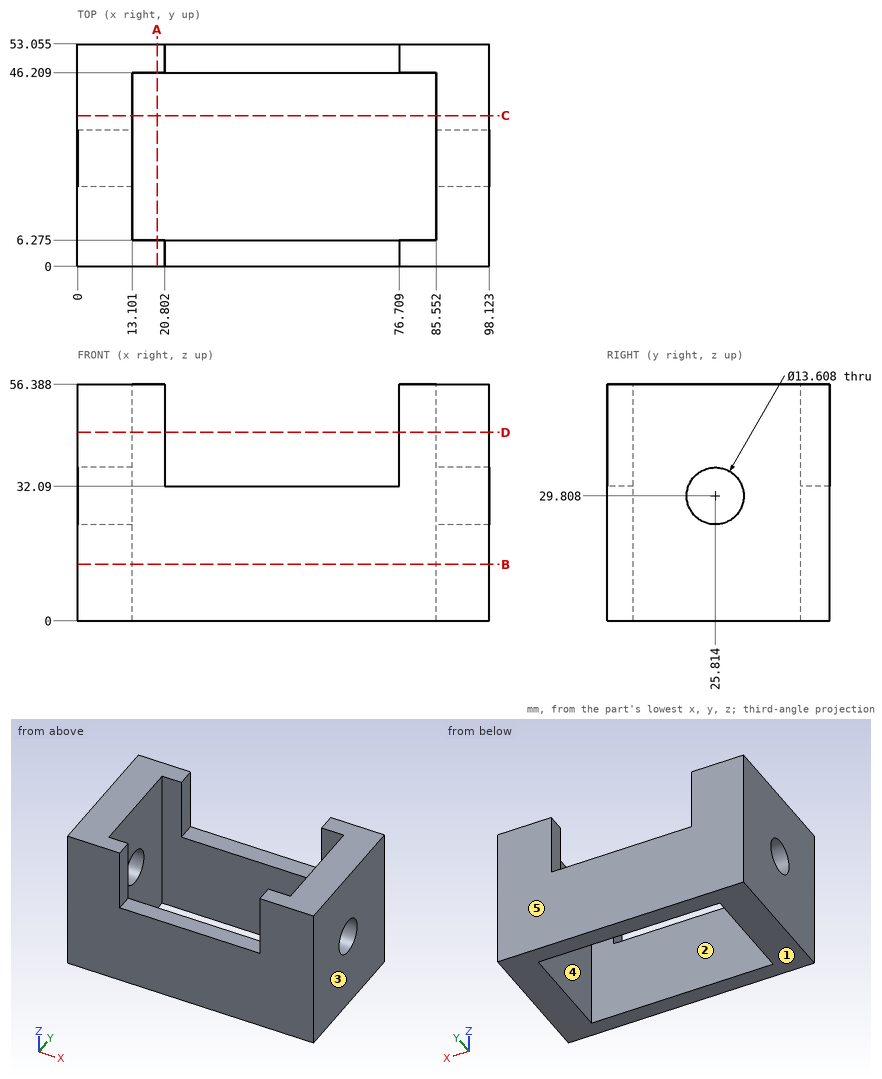
Source: three-view drawing plus pictorial views. Frame: mm from the lowest corner of the part. A direction names the side the tool comes from. Give positions to 0.01 mm unless a question says otherwise; leave off trailing zeros. Write each loop counter-clockwise with the first axis right and the second up, starting at its lowest first coordinate (ties: lowest second). Pieces come first, ordered by that corner, then holes. Notation, with made-up numbers: (-15, 33) -> (4, 33) arc R30 cw to (4, 68) -> close; hole circle Ø2 at (-39, 74.25). An arc over 180 degrees is marked (long way). Write item = value, one per line.
Q1. Mould query, pull axis X, two halves, no side actions, for the marked faces 1, 2 and 3. Classes: +X half, -X half, draft (parallel to the pull), parting line (faces both ways), or undercut.
Here are the results:
face_1 = draft
face_2 = undercut
face_3 = +X half
Q2. Reachability of the marked faces 4 and 5 from +Z, -Z, +X, -X, +Y, -Y: full face, straight path, thin tool, end or side. Return the list, or none.
Here are the results:
face_4 = +Z, -Z
face_5 = +Z, -Z, +X, -X, +Y
Q3. First-contact query: pin 1 (6 mm diameter, centred on x = 37, z = 37.5, fed in from -Y); pin 2 (7.5 mm diameter, centred on x = 54, y = 50.5, fed in from +Z). Flat tips, straight axial feed; report the tip coordinate or a pass-through.
Here are the results:
pin_1 = through
pin_2 = 32.09
Q4. Cut plane C-C on y = 36. Return loops of the section in (x, z).
Here are the results:
outline = (0, 0) -> (13.1, 0) -> (13.1, 56.39) -> (0, 56.39) -> close; (85.55, 0) -> (98.12, 0) -> (98.12, 56.39) -> (85.55, 56.39) -> close
Q5. Line query: line 1 (Y direction, x = 24, z = 15) (1 decimal); line 2 (X direction, y = 19.5, z = 35); line 3 (X direction, y = 49.5, z = 51). Output: solid intervals per line, ascending. Write a range as from..to.
Here are the results:
line_1 = 0..6.3, 46.2..53.1
line_2 = 0..13.1, 85.55..98.12
line_3 = 0..20.8, 76.71..98.12
Q6. Cut plane D-D on z = 45. Return loops of the section in (x, y) (1 decimal).
Here are the results:
outline = (0, 0) -> (20.8, 0) -> (20.8, 6.3) -> (13.1, 6.3) -> (13.1, 46.2) -> (20.8, 46.2) -> (20.8, 53.1) -> (0, 53.1) -> close; (76.7, 0) -> (98.1, 0) -> (98.1, 53.1) -> (76.7, 53.1) -> (76.7, 46.2) -> (85.6, 46.2) -> (85.6, 6.3) -> (76.7, 6.3) -> close
Q7. Cut plane A-A on x = 19. Return loops of the section in (y, z) (1 decimal).
Here are the results:
outline = (0, 0) -> (6.3, 0) -> (6.3, 56.4) -> (0, 56.4) -> close; (46.2, 0) -> (53.1, 0) -> (53.1, 56.4) -> (46.2, 56.4) -> close
Q8. Cut plane B-B on z = 13.5. Return loops of the section in (x, y) (1 decimal).
Here are the results:
outline = (0, 0) -> (98.1, 0) -> (98.1, 53.1) -> (0, 53.1) -> close; hole (13.1, 6.3) -> (85.6, 6.3) -> (85.6, 46.2) -> (13.1, 46.2) -> close
